Geometry: final body of the model. Coordinates: model frame, mm. Face numbers are marked on the shaded views. A direction names the side the tool comes from. Coordinates: 2 decimals unless noted, no trailing zeros. Write each loop counter-clockwise with the first axis right and the second up, starting at its lowest first coordinate (ties: lowest second). Pieces come first, ordered by that corner, then holes. Notation, with made-up numbers: (22.5, 48) - (45.5, 48) arc R17 ccw to (45.5, 68) - close; hole circle Ø7 at (6.5, 12). An arc over 180 degrees is marked (long way). Answer as a JSON object with one key per item and string values. Group by question number.
Item 1: Line query: line 1 along Z through (x, y) = (8, 9); line 2 along Z through (x, y) = (14.5, 20); line 3 along Y through (x, z) = (-28.5, 9). Output: solid intervals per line, ascending. Write a range as from..to.
Item 2: Mould query, pull axis X, two halves, no side actions, for the marked faces 4, 5 and 6. Classes: pulls with the +X half, pulls with the -X half, needs draft (parallel to the pull), parting line crosses it, or undercut.
Item 3: Set-up query: the marked faces 1, 2 and 3. Return all of +Z, -Z, +X, -X, +Y, -Y with unobstructed straight access to the full face (end or side cutting, diameter ignored); none if empty.
Item 4: First-contact query: pin 1 Ø4 at (x, z) = (1, 13) entering from -Y; pin 2 Ø2 at (x, y) = (10, 10.5) entering from +Z; pin 3 Ø12 at (x, y) = (27.5, 19.5) entering from +Z. Flat tips, straight axial feed; report the tip coordinate or a pass-through.
Item 5: Section B-B on x = 1. Return loops of the section in (y, z), and give its area (3 significant figures).
Item 6: Section C-C on y = 16. Return loops of the section in (x, z).
Item 7: Section D-D on z = 20. Return loops of the section in (x, y), and give its area (3 significant figures).
Item 8: Section A-A on z = 5. Return loops of the section in (x, y).
```python
from build123d import *

# Parameters (mm, degrees)
F1_DEPTH = 15.85
F3_DEPTH = 1.6
F5_DEPTH = 25.4


with BuildPart() as f1:
    # F0 (on Top) → F1 (new body)
    with BuildSketch(Plane.XY):
        Polygon((-16.495027, 4.112672), (0, 0), (16.495027, 4.112672), (16.132145, 5.568116), (40.777656, 11.712932), (36.89481, 27.286178), (12.249298, 21.141362), (11.886415, 22.596806), (5.849207, 21.091561), (0, 26.940768), (-5.849207, 21.091561), (-11.886415, 22.596806), (-12.249298, 21.141362), (-36.89481, 27.286178), (-40.777656, 11.712932), (-16.132145, 5.568116), align=None)
    extrude(amount=F1_DEPTH)

    # F2 (on face) → F3 (join)
    with BuildSketch(Plane.XY.offset(15.85)):
        Polygon((-16.132145, 5.568116), (-16.495027, 4.112672), (0, 0), (16.495027, 4.112672), (16.132145, 5.568116), (12.249298, 21.141362), (11.886415, 22.596806), (5.849207, 21.091561), (0, 26.940768), (-5.849207, 21.091561), (-11.886415, 22.596806), (-12.249298, 21.141362), align=None)
    extrude(amount=F3_DEPTH)

    # F4 (on face) → F5 (join)
    with BuildSketch(Plane.XY.offset(17.45)):
        Polygon((-11.349064, 13.470384), (0, 2.12132), (11.349064, 13.470384), (0, 24.819448), align=None)
    extrude(amount=F5_DEPTH)


solid = f1.part
```
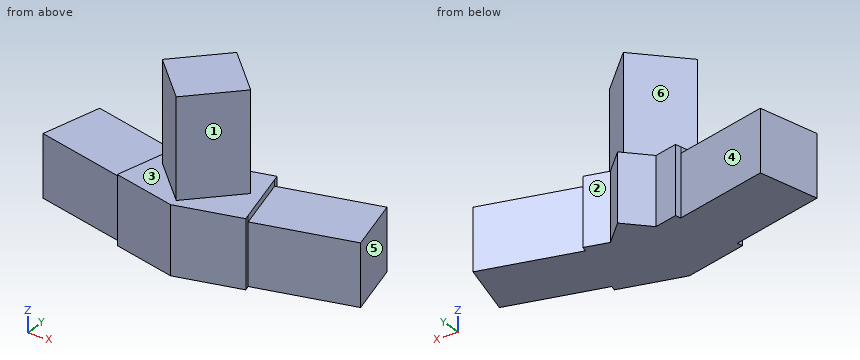
Checks:
{
 "1": {"line 1": "0..17.45", "line 2": "0..15.85", "line 3": "8.65..25.19"},
 "2": {"face 4": "undercut", "face 5": "pulls with the +X half", "face 6": "pulls with the -X half"},
 "3": {"face 1": "+Z, +X, -Y", "face 2": "+Z, -Z, +Y", "face 3": "+Z"},
 "4": {"pin 1": "y = 0", "pin 2": "z = 17.45", "pin 3": "z = 15.85"},
 "5": {"outline": "(0.25, 0) - (25.94, 0) - (25.94, 17.45) - (23.82, 17.45) - (23.82, 42.85) - (3.12, 42.85) - (3.12, 17.45) - (0.25, 17.45) - close", "area": "974 mm^2"},
 "6": {"outline": "(-39.71, 0) - (39.71, 0) - (39.71, 15.85) - (13.53, 15.85) - (13.53, 17.45) - (8.82, 17.45) - (8.82, 42.85) - (-8.82, 42.85) - (-8.82, 17.45) - (-13.53, 17.45) - (-13.53, 15.85) - (-39.71, 15.85) - close"},
 "7": {"outline": "(-11.35, 13.47) - (0, 2.12) - (11.35, 13.47) - (0, 24.82) - close", "area": "258 mm^2"},
 "8": {"outline": "(-40.78, 11.71) - (-16.13, 5.57) - (-16.5, 4.11) - (0, 0) - (16.5, 4.11) - (16.13, 5.57) - (40.78, 11.71) - (36.89, 27.29) - (12.25, 21.14) - (11.89, 22.6) - (5.85, 21.09) - (0, 26.94) - (-5.85, 21.09) - (-11.89, 22.6) - (-12.25, 21.14) - (-36.89, 27.29) - close"}
}
